from build123d import *

# Parameters (mm, degrees)
SKETCH_1_R               = 16.5
EXTRUDE_1_DEPTH          = 6.5
EXTRUDE_START            = 4
SKETCH_2_R               = 16.5
SKETCH_2_R_2             = 16
EXTRUDE_2_DEPTH          = 4
CUT_EXTRUDE_START        = -4
SKETCH_4_R               = 16
CUT_EXTRUDE_2_DEPTH      = 4
SKETCH_5_R               = 20
SKETCH_5_R_2             = 16.5
EXTRUDE_3_DEPTH          = 3
EXTRUDE_START_2          = -3
SKETCH_6_R               = 20
SKETCH_6_R_2             = 16.5
EXTRUDE_4_DEPTH          = 3
CHAMFER_1_SIZE           = 1
SKETCH_7_R               = 0.75
CUT_EXTRUDE_3_DEPTH      = 33.445844482
PATTERN_CIRCULAR_1_COUNT = 3
CHAMFER_2_SIZE           = 0.5


with BuildPart() as part:
    # 草图1 → 凸台-拉伸1 (new body)
    with BuildSketch(Plane.XY.offset(13.616672725)):
        with Locations(Location((0.173765051, -3.140916746, 0), (0, 0, 180))):
            Circle(SKETCH_1_R)
        with BuildLine():
            ThreePointArc((-4.541092987, 11.624587434), (-6.265167651, 10.958379182), (-7.897683054, 10.091684113))
            ThreePointArc((-7.897683054, 10.091684113), (-8.333327501, 9.530083474), (-8.285825063, 8.820911505))
            ThreePointArc((-8.285825063, 8.820911505), (-8.666854858, 7.061702508), (-10.462383837, 6.934912591))
            ThreePointArc((-10.462383837, 6.934912591), (-11.157577156, 7.082857217), (-11.77546018, 6.731571106))
            ThreePointArc((-11.77546018, 6.731571106), (-12.865664708, 5.239015925), (-13.770453328, 3.627301174))
            ThreePointArc((-13.770453328, 3.627301174), (-13.833316529, 2.919325482), (-13.409947623, 2.348413815))
            ThreePointArc((-13.409947623, 2.348413815), (-12.779390093, 0.662472772), (-14.221337386, -0.414925949))
            ThreePointArc((-14.221337386, -0.414925949), (-14.886156125, -0.666316895), (-15.216032792, -1.295890359))
            ThreePointArc((-15.216032792, -1.295890359), (-15.326234949, -3.140916746), (-15.216032792, -4.985943132))
            ThreePointArc((-15.216032792, -4.985943132), (-14.886156125, -5.615516597), (-14.221337386, -5.866907543))
            ThreePointArc((-14.221337386, -5.866907543), (-12.779390093, -6.944306263), (-13.409947623, -8.630247307))
            ThreePointArc((-13.409947623, -8.630247307), (-13.833316529, -9.201158974), (-13.770453328, -9.909134666))
            ThreePointArc((-13.770453328, -9.909134666), (-12.865664708, -11.520849416), (-11.77546018, -13.013404598))
            ThreePointArc((-11.77546018, -13.013404598), (-11.157577156, -13.364690708), (-10.462383837, -13.216746083))
            ThreePointArc((-10.462383837, -13.216746083), (-8.666854858, -13.343536), (-8.285825063, -15.102744997))
            ThreePointArc((-8.285825063, -15.102744997), (-8.333327501, -15.811916965), (-7.897683054, -16.373517605))
            ThreePointArc((-7.897683054, -16.373517605), (-6.265167651, -17.240212674), (-4.541092987, -17.906420926))
            ThreePointArc((-4.541092987, -17.906420926), (-3.8313771, -17.867888824), (-3.326528168, -17.367580001))
            ThreePointArc((-3.326528168, -17.367580001), (-1.747485266, -16.503506211), (-0.475842415, -17.777446736))
            ThreePointArc((-0.475842415, -17.777446736), (-0.132396696, -18.399721916), (0.537714963, -18.636643268))
            ThreePointArc((0.537714963, -18.636643268), (2.379645044, -18.483149095), (4.19020832, -18.111494005))
            ThreePointArc((4.19020832, -18.111494005), (4.76642729, -17.695377361), (4.920645867, -17.001548857))
            ThreePointArc((4.920645867, -17.001548857), (5.781867726, -15.420948683), (7.540386014, -15.805153619))
            ThreePointArc((7.540386014, -15.805153619), (8.165738301, -16.142964039), (8.857561455, -15.979985248))
            ThreePointArc((8.857561455, -15.979985248), (10.324106427, -14.855035148), (11.646317267, -13.563514581))
            ThreePointArc((11.646317267, -13.563514581), (11.906093869, -12.901927489), (11.660718782, -12.234864952))
            ThreePointArc((11.660718782, -12.234864952), (11.530687744, -10.439567781), (13.217764337, -9.812054777))
            ThreePointArc((13.217764337, -9.812054777), (13.926478259, -9.758148014), (14.420363945, -9.247013695))
            ThreePointArc((14.420363945, -9.247013695), (15.045906142, -7.507771377), (15.459971947, -5.706433987))
            ThreePointArc((15.459971947, -5.706433987), (15.320828945, -5.009425675), (14.753765051, -4.580916746))
            ThreePointArc((14.753765051, -4.580916746), (13.673765051, -3.140916746), (14.753765051, -1.700916746))
            ThreePointArc((14.753765051, -1.700916746), (15.320828945, -1.272407817), (15.459971947, -0.575399504))
            ThreePointArc((15.459971947, -0.575399504), (15.045906142, 1.225937885), (14.420363945, 2.965180204))
            ThreePointArc((14.420363945, 2.965180204), (13.926478259, 3.476314523), (13.217764337, 3.530221285))
            ThreePointArc((13.217764337, 3.530221285), (11.530687744, 4.15773429), (11.660718782, 5.95303146))
            ThreePointArc((11.660718782, 5.95303146), (11.906093869, 6.620093998), (11.646317267, 7.281681089))
            ThreePointArc((11.646317267, 7.281681089), (10.324106427, 8.573201657), (8.857561455, 9.698151757))
            ThreePointArc((8.857561455, 9.698151757), (8.165738301, 9.861130547), (7.540386014, 9.523320128))
            ThreePointArc((7.540386014, 9.523320128), (5.781867726, 9.139115191), (4.920645867, 10.719715365))
            ThreePointArc((4.920645867, 10.719715365), (4.76642729, 11.413543869), (4.19020832, 11.829660513))
            ThreePointArc((4.19020832, 11.829660513), (2.379645044, 12.201315603), (0.537714963, 12.354809777))
            ThreePointArc((0.537714963, 12.354809777), (-0.132396696, 12.117888425), (-0.475842415, 11.495613244))
            ThreePointArc((-0.475842415, 11.495613244), (-1.747485266, 10.22167272), (-3.326528168, 11.08574651))
            ThreePointArc((-3.326528168, 11.08574651), (-3.8313771, 11.586055332), (-4.541092987, 11.624587434))
        make_face(mode=Mode.SUBTRACT)
    extrude(amount=EXTRUDE_1_DEPTH)

    # 草图2 → 凸台-拉伸2 (add)
    with BuildSketch(Plane(origin=(0, 0, 13.616672725), x_dir=(-1, 0, 0), z_dir=(0, 0, -1)).offset(EXTRUDE_START)):
        with Locations((-0.173765051, -3.140916746)):
            Circle(SKETCH_2_R)
        with Locations((-0.173765051, -3.140916746)):
            Circle(SKETCH_2_R_2, mode=Mode.SUBTRACT)
    extrude(amount=-EXTRUDE_2_DEPTH)

    # 草图4 → 切除-拉伸2 (cut)
    with BuildSketch(Plane.XY.offset(20.116672725).offset(CUT_EXTRUDE_START)):
        with Locations(Location((0.173765051, -3.140916746, 0), (0, 0, 180))):
            Circle(SKETCH_4_R)
    extrude(amount=CUT_EXTRUDE_2_DEPTH, mode=Mode.SUBTRACT)

    # 草图5 → 凸台-拉伸3 (add)
    with BuildSketch(Plane(origin=(0, 0, 9.616672725), x_dir=(-1, 0, 0), z_dir=(0, 0, -1))):
        with Locations((-0.173765051, -3.140916746)):
            Circle(SKETCH_5_R)
        with Locations((-0.173765051, -3.140916746)):
            Circle(SKETCH_5_R_2, mode=Mode.SUBTRACT)
    extrude(amount=-EXTRUDE_3_DEPTH)

    # 草图6 → 凸台-拉伸4 (add)
    with BuildSketch(Plane.XY.offset(20.116672725).offset(EXTRUDE_START_2)):
        with Locations(Location((0.173765051, -3.140916746, 0), (0, 0, 180))):
            Circle(SKETCH_6_R)
        with Locations(Location((0.173765051, -3.140916746, 0), (0, 0, 180))):
            Circle(SKETCH_6_R_2, mode=Mode.SUBTRACT)
    extrude(amount=EXTRUDE_4_DEPTH)

    # 倒角1
    chamfer_1_edges = [part.edges().sort_by_distance(p)[0] for p in [
        (20.173765051, -3.140916746, 12.616672725),
        (20.173765051, -3.140916746, 9.616672725),
        (20.173765051, -3.140916746, 17.116672725),
        (20.173765051, -3.140916746, 20.116672725),
    ]]
    chamfer(chamfer_1_edges, length=CHAMFER_1_SIZE)

    # 草图7 → 切除-拉伸3 (cut, through all)
    with BuildSketch(Plane.XY.offset(20.116672725)):
        with Locations((17.750861301, -0.675711568)):
            Circle(SKETCH_7_R)
    cut_extrude_3 = extrude(amount=-CUT_EXTRUDE_3_DEPTH, mode=Mode.SUBTRACT)

    # 阵列(圆周)1: 切除-拉伸3 ×3 about axis
    pattern_circular_1_axis = Axis((0.173765051, -3.140916746, 0), (0, 0, 1))
    for i in range(1, PATTERN_CIRCULAR_1_COUNT):
        add(cut_extrude_3.rotate(pattern_circular_1_axis, i * 360 / PATTERN_CIRCULAR_1_COUNT), mode=Mode.SUBTRACT)

    # 倒角2
    chamfer_2_edges = [part.edges().sort_by_distance(p)[0] for p in [
        (16.173765051, -3.140916746, 20.116672725),
    ]]
    chamfer(chamfer_2_edges, length=CHAMFER_2_SIZE)


solid = part.part
Here's how the part is built. I have some questions about the finished solid (model axes, mm). A direction names the side the tool comes from. Coordinates: 2 decimals unless noted, no trailing zeros. Use one line per item in the form item = value.
1) On a 3-axis mill with a long thin cutter (end or side, diameter ignored), from which of +Z, -Z, +X, -X, +Y, -Y can I reach the whole of each face in a straight line? I mean faces 1 (the flat face through (6, -19, 20.117)), 2 (the cylindrical face through (-15.326, -3.115, 14.849)), 3 (the cylindrical face through (-15.087, 1.665, 11.589)), 4 (the cylindrical face through (3.64, 12.48, 17.84)). Say none if no direction works.
Solved:
face_1 = +Z, +X, -X, +Y, -Y
face_2 = +Z, -Z
face_3 = -Z
face_4 = +Z
2) I'm going to push flat-ended pins straight in: P1, Ø19, axis at x = -5, y = -1, coming from the -Z side; P2, Ø1, axis at y = -12, z = 11.5, coming from the +X side; P3, Ø0.9, axis at x = -6.48, y = -19.6, coming from the +Z side; P4, Ø3, axis at x = 10.5, z = 17, coming from the -Y side. Where does each tip first touch, or does it pass through?
Solved:
P1 = 13.62
P2 = 18.34
P3 = through
P4 = -20.83
3) I need wall thicknesses on line 1 (X direction, y = -3.5, z = 16.75); line 2 (Z direction, x = -9.5, y = -18); line 3 (X direction, y = -3, z = 19). Which ranges of each line are inside material? Lowest first, please.
Solved:
line_1 = -16.32 to -15.82, 16.17 to 16.67
line_2 = 9.62 to 12.62, 17.12 to 20.12
line_3 = -19.83 to -15.83, 16.17 to 20.17
